Design review of the part shown in the three views and the two pictorial views. Dimensions are in mm from the part's minimum x, y and z. Give positions to 0.01 mm unless a question says otherwise; leave off trailing zeros. Loops run counter-clockwise (first coordinate to the right, second up) from the corner with the lowest first, then second, coordinate; pieces in that order, holes last. Notation, with made-up numbers: (30.25, 14) - (39.25, 14) arc R5 cw to (39.25, 21) - close; hole circle Ø1 at (-21.5, -22). An arc over 180 degrees is marked (long way). Answer as a JSON object with one key per item and string values.
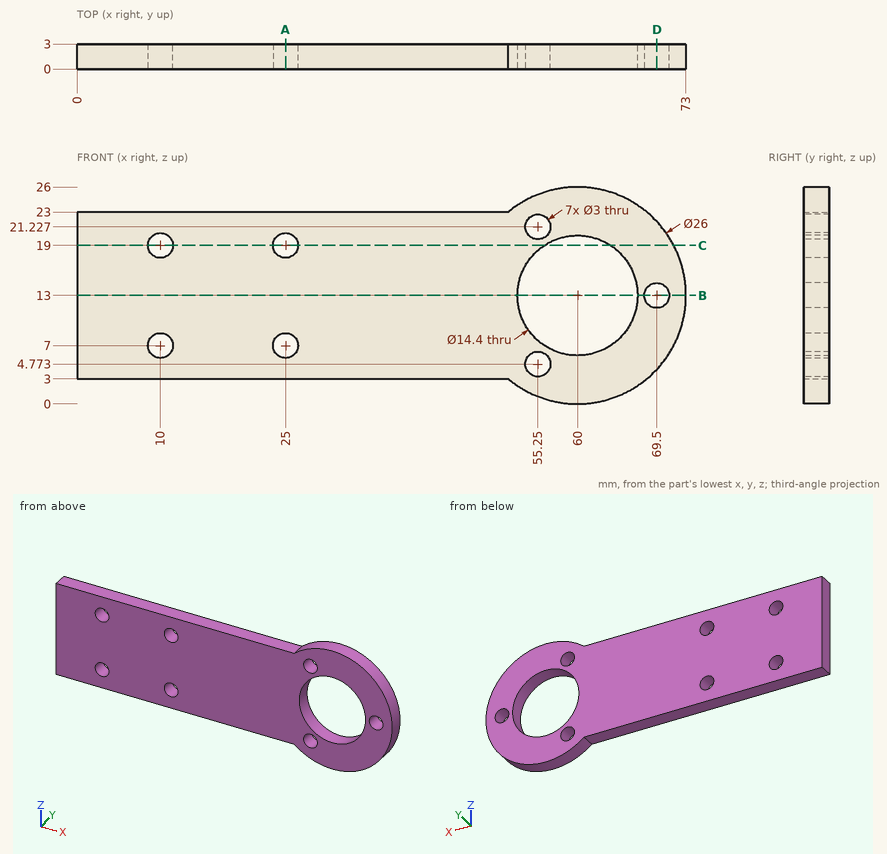
Q1. Consider section C-C, the plane z = 19. State the section outline as (x, y) points, plus the area to 3 significant figures.
Results:
{"outline": "(0, 0) - (8.5, 0) - (8.5, 3) - (0, 3) - close; (11.5, 0) - (23.5, 0) - (23.5, 3) - (11.5, 3) - close; (26.5, 0) - (56.02, 0) - (56.02, 3) - (26.5, 3) - close; (63.98, 0) - (71.53, 0) - (71.53, 3) - (63.98, 3) - close", "area": "173 mm^2"}
Q2. Consider section D-D, the plane x = 69.5. State the section outline as (y, z) points.
Results:
{"outline": "(0, 4.13) - (3, 4.13) - (3, 11.5) - (0, 11.5) - close; (0, 14.5) - (3, 14.5) - (3, 21.87) - (0, 21.87) - close"}
Q3. Consider section B-B, the plane z = 13. State the section outline as (x, y) points, plus the area to 3 significant figures.
Results:
{"outline": "(0, 0) - (52.8, 0) - (52.8, 3) - (0, 3) - close; (67.2, 0) - (68, 0) - (68, 3) - (67.2, 3) - close; (71, 0) - (73, 0) - (73, 3) - (71, 3) - close", "area": "167 mm^2"}
Q4. Clearance check with flat-ended pins moving along their axes: pin 1 Ø1 at (y, z) = (1, 16) entering from +X; pin 2 Ø0.9 at (x, y) = (23.5, 2) entering from +Z. State where each tip first meets the part, or that it passes through.
Results:
{"pin 1": "stops at x = 72.76", "pin 2": "stops at z = 23"}
Q5. Consider section A-A, the plane x = 25. State the section outline as (y, z) points, plus the area to 3 significant figures.
Results:
{"outline": "(0, 3) - (3, 3) - (3, 5.5) - (0, 5.5) - close; (0, 8.5) - (3, 8.5) - (3, 17.5) - (0, 17.5) - close; (0, 20.5) - (3, 20.5) - (3, 23) - (0, 23) - close", "area": "42.0 mm^2"}
Q6. To check wall thickness, follow probe 1 along Z at (x, y) = (25, 1.05); probe 2 along Z at (x, y) = (26, 0.75); probe 3 along X at (y, z) = (0.6, 14). State the ranges of each line that lie inside material, in increasing order. Write a range as [from, to].
Results:
{"probe 1": "z = [3, 5.5], [8.5, 17.5], [20.5, 23]", "probe 2": "z = [3, 5.88], [8.12, 17.88], [20.12, 23]", "probe 3": "x = [0, 52.87], [67.13, 68.38], [70.62, 72.96]"}
